from build123d import *

# Parameters (mm, degrees)
SKETCH_R  = 2.2
PAD_DEPTH = 2


with BuildPart() as part:
    # Sketch → Pad (new body)
    with BuildSketch(Plane.XY):
        with BuildLine():
            ThreePointArc((-4, 0), (0, -4), (4, 0))
            Line((2.692664, 14.94292), (4, 0))
            ThreePointArc((2.692664, 14.94292), (2.399771, 15.650027), (1.692664, 15.94292))
            Line((1.692664, 15.94292), (0, 15.94292))
            Line((-1.692664, 15.94292), (0, 15.94292))
            ThreePointArc((-1.692664, 15.94292), (-2.399771, 15.650027), (-2.692664, 14.94292))
            Line((-4, 0), (-2.692664, 14.94292))
        make_face()
        Circle(SKETCH_R, mode=Mode.SUBTRACT)
    extrude(amount=PAD_DEPTH)


solid = part.part
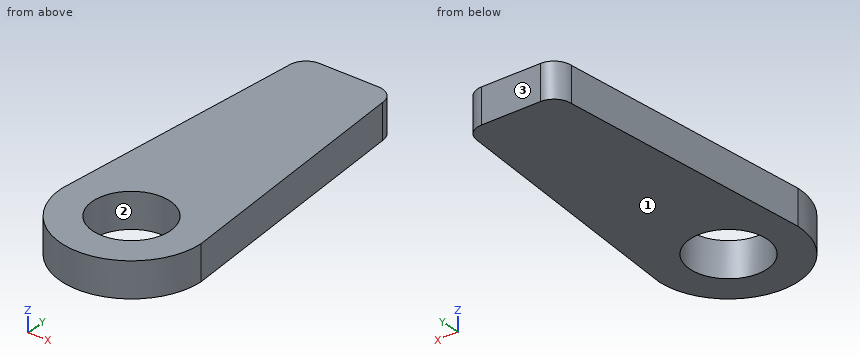
Could you check a few things on this model? Use its own coordinates, in mm. Face numbers are marked on the shaded views. Give positions to 0.01 mm unless a question says otherwise; leave off trailing zeros. Order: outer loops, then holes, each group sorted by start corner. A loop starts at its lowest first (then second) coordinate and runs counter-clockwise, first axis right, second up. Notation, with made-up numbers: (52.5, 9.5) - (80.5, 9.5) arc R13 cw to (80.5, 18.5) - close; hole circle Ø11 at (64, 40). An arc over 180 degrees is marked (long way). One line per item, written item: value. Start each with the question number.
1. Imagine slicing it at D-D on y = -2.75. List the corners of the cut face in (x, z) for me.
2. Imagine slicing it at B-B on z = 0.7. List the corners of the cut face in (x, y) for me.
3. If I drill on probe 1 along Y at (x, z) = (0, 0.8); probe 2 along Y at (x, z) = (-1, 1.6); probe 3 along X at (y, z) = (-1.5, 1.25), over which ranges is the centre line in solid material (lowest first)?
4. Imagine slicing it at C-C on y = -0.5. List the corners of the cut face in (x, z) for me.
5. Imagine slicing it at A-A on x = 0. List the corners of the cut face in (y, z) for me.
6. Thinking about a two-plate mould opening in Y: for the marked faces 1, 2 and 3, which applies, +Y half, -Y half, draft (parallel to the pull), parting line (faces both ways), or undercut?
Values:
1. outline: (-2.9, 0) - (2.9, 0) - (2.9, 2) - (-2.9, 2) - close
2. outline: (-4, 0) arc R4 ccw to (4, 0) - (2.69, 14.94) arc R1 ccw to (1.69, 15.94) - (-1.69, 15.94) arc R1 ccw to (-2.69, 14.94) - close; hole circle Ø4.4 at (0, 0)
3. probe 1: -4 to -2.2, 2.2 to 15.94
3. probe 2: -3.87 to -1.96, 1.96 to 15.94
3. probe 3: -3.71 to -1.61, 1.61 to 3.71
4. outline: (-3.97, 0) - (-2.14, 0) - (-2.14, 2) - (-3.97, 2) - close; (2.14, 0) - (3.97, 0) - (3.97, 2) - (2.14, 2) - close
5. outline: (-4, 0) - (-2.2, 0) - (-2.2, 2) - (-4, 2) - close; (2.2, 0) - (15.94, 0) - (15.94, 2) - (2.2, 2) - close
6. face 1: draft
6. face 2: undercut
6. face 3: +Y half
